Work out the finished part from the listing and answer in its coordinate system (mm). Face numbers are marked on the shaded views. A direction names the side the tool comes from. Give positions to 0.01 mm unless a question says otherwise; leave off trailing zeros. Write each loop counter-clockwise with the first axis right and the second up, starting at its lowest first coordinate (ties: lowest second). Pieces come first, ordered by that corner, then holes.
1) Straight lines are drawn through the part: probe 1 along Y at (x, z) = (6.75, 6.75); probe 2 along Z at (x, y) = (7.25, -1.25). For each, find the intervals that lie inside material, in ascending order.
2) Given pin 1 Ø4 at (y, z) = (5.5, 10.5) entering from -X, flat-ended and moving along its own axis, determine where the tip first touches the part or whether it passes through.
3) Find section C-C (x = 7.25). Determine the outline of the cut face in (y, z), plus the area to 3 significant figures.
4) Find section A-A (z = 8). Determine the outline of the cut face in (x, y), plus the area to 3 significant figures.
5) Find section D-D (z = -0.25). Determine the outline of the cut face in (x, y).
6) Determine the mould class of the marked faces 3, 4, 5 and 6 for opening direction Y: pulls with the +Y half, pulls with the -Y half, needs draft (parallel to the pull), parting line crosses it, or undercut.
7) Find section B-B (y = 1.75). Determine the outline of the cut face in (x, z).
8) A tool of negligible diameter and unlimited length cuts with its end or side. For the marked faces 1 and 2, from which of +Z, -Z, +X, -X, +Y, -Y can it reach the whole face along a straight path? Write none if from no direction.
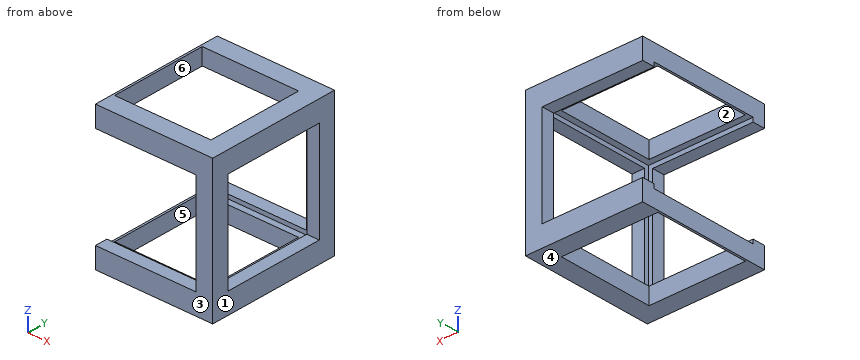
```python
from build123d import *

# Parameters (mm, degrees)
F0_W      = 16
F0_H      = 16
F0_W_2    = 13
F0_H_2    = 13
F1_DEPTH  = 13
F2_W      = 16
F2_H      = 16
F2_W_2    = 11.5
F2_H_2    = 11.5
F3_DEPTH  = 2
F4_W      = 16
F4_H      = 16
F4_W_2    = 11.5
F4_H_2    = 11.5
F5_DEPTH  = 2
F6_W      = 12
F6_H      = 12
F7_DEPTH  = 16.001
F8_W      = 12
F8_H      = 12
F9_DEPTH  = 1.5
F10_W     = 16
F10_H     = 17
F11_DEPTH = 2


with BuildPart() as f1:
    # F0 (on Top) → F1 (new body)
    with BuildSketch(Plane.XY):
        Rectangle(F0_W, F0_H)
        Rectangle(F0_W_2, F0_H_2, mode=Mode.SUBTRACT)
    extrude(amount=F1_DEPTH)

    # F2 (on face) → F3 (join)
    with BuildSketch(Plane(origin=(0, 0, 0), x_dir=(1, 0, 0), z_dir=(0, 0, -1))):
        Rectangle(F2_W, F2_H)
        Rectangle(F2_W_2, F2_H_2, mode=Mode.SUBTRACT)
    extrude(amount=F3_DEPTH)

    # F4 (on face) → F5 (join)
    with BuildSketch(Plane.XY.offset(13)):
        Rectangle(F4_W, F4_H)
        Rectangle(F4_W_2, F4_H_2, mode=Mode.SUBTRACT)
    extrude(amount=F5_DEPTH)

    # F6 (on face) → F7 (cut, through all)
    with BuildSketch(Plane(origin=(0, 8, 0), x_dir=(-1, 0, 0), z_dir=(0, 1, 0))):
        with Locations((0, 6.5)):
            Rectangle(F6_W, F6_H)
    extrude(amount=-F7_DEPTH, mode=Mode.SUBTRACT)

    # F8 (on face) → F9 (cut, through all)
    with BuildSketch(Plane.YZ.offset(8)):
        with Locations((0, 6.5)):
            Rectangle(F8_W, F8_H)
    extrude(amount=-F9_DEPTH, mode=Mode.SUBTRACT)

    # F10 (on face) → F11 (cut)
    with BuildSketch(Plane(origin=(-8, 0, 0), x_dir=(0, -1, 0), z_dir=(-1, 0, 0))):
        with Locations((0, 6.5)):
            Rectangle(F10_W, F10_H)
    extrude(amount=-F11_DEPTH, mode=Mode.SUBTRACT)


solid = f1.part
```
Results:
1. probe 1: y = -8 to -6, 6 to 8
1. probe 2: z = -2 to 0.5, 12.5 to 15
2. pin 1: stops at x = 6
3. outline: (-8, -2) - (8, -2) - (8, 15) - (-8, 15) - close; hole (-6, 0.5) - (6, 0.5) - (6, 12.5) - (-6, 12.5) - close
3. area: 128 mm2
4. outline: (6, -8) - (8, -8) - (8, -6) - (6.5, -6) - (6.5, -6.5) - (6, -6.5) - close; (6, 6.5) - (6.5, 6.5) - (6.5, 6) - (8, 6) - (8, 8) - (6, 8) - close
4. area: 7.50 mm2
5. outline: (-6, -8) - (8, -8) - (8, 8) - (-6, 8) - close; hole (-5.75, -5.75) - (5.75, -5.75) - (5.75, 5.75) - (-5.75, 5.75) - close
6. face 3: pulls with the -Y half
6. face 4: needs draft
6. face 5: undercut
6. face 6: undercut
7. outline: (-6, -2) - (-5.75, -2) - (-5.75, 0) - (-6, 0) - close; (-6, 13) - (-5.75, 13) - (-5.75, 15) - (-6, 15) - close; (5.75, -2) - (8, -2) - (8, 0.5) - (6.5, 0.5) - (6.5, 0) - (5.75, 0) - close; (5.75, 13) - (6.5, 13) - (6.5, 12.5) - (8, 12.5) - (8, 15) - (5.75, 15) - close
8. face 1: +Z, -Z, +X, +Y, -Y
8. face 2: +Z, -Z
